Model file for the job. Use its own axes, mm. Round coordinates to 2 decimals unless told otherwise and drop trailing zeros. Order: outer loops, then holes, each group sorted by start corner. A loop starts at its lowest first (then second) coordinate and runs counter-clockwise, first axis right, second up. Notation, with made-up numbers: (4, -17.75) - (23, -17.75) arc R21 cw to (23, -4.75) - close; hole circle Ø10 at (-2.5, 31). An arc over 180 degrees is marked (long way). Put each result on its own line as item: value. Start each with the question number.
Item 1: Saw through at B-B on x = -4.5. List the corners of the cut face in (y, z), plus the area to 3 significant figures.
Item 2: Saw through at A-A on y = 0. List the corners of the cut face in (x, z).
Item 3: Probe probe 1 along Y at (x, z) = (0, 1.05); probe 2 along X at (y, z) = (11, 2.2); probe 3 along X at (y, z) = (-3, 0.7). List the from-to ranges inside material, lowest first.
Item 4: Mould opens along Y. For faces 1 (the face through (63.5, 0, 1)), 2 (the face through (31, 19.939, 1)), 3 (the face through (-3.909, -17.605, 1.288)) say: pulls with the +Y half, pulls with the -Y half, needs draft (parallel to the pull), parting line crosses it, or undercut.
Item 5: Saw through at C-C on z = 1.8. List the corners of the cut face in (x, y).
```python
from build123d import *

# Parameters (mm, degrees)
SKETCH1_R           = 19.939
BOSS_EXTRUDE1_DEPTH = 2.54
SKETCH3_W           = 2.54
SKETCH3_H           = 39.878
BOSS_EXTRUDE2_DEPTH = 63.5
SKETCH2_R           = 18.034
CUT_EXTRUDE1_DEPTH  = 2.54


with BuildPart() as part:
    # Sketch1 → Boss-Extrude1 (new body)
    with BuildSketch(Plane.XY):
        Circle(SKETCH1_R)
    extrude(amount=BOSS_EXTRUDE1_DEPTH)

    # Sketch3 → Boss-Extrude2 (add)
    with BuildSketch(Plane(origin=(0, 0, 0), x_dir=(0, 0, -1), z_dir=(1, 0, 0))):
        with Locations((-1.27, 0)):
            Rectangle(SKETCH3_W, SKETCH3_H)
    extrude(amount=BOSS_EXTRUDE2_DEPTH)

    # Sketch2 → Cut-Extrude1 (cut)
    with BuildSketch(Plane.XY.offset(2.54)):
        Circle(SKETCH2_R)
    extrude(amount=-CUT_EXTRUDE1_DEPTH, mode=Mode.SUBTRACT)


solid = part.part
```
Results found:
1. outline: (-19.42, 0) - (-17.46, 0) - (-17.46, 2.54) - (-19.42, 2.54) - close; (17.46, 0) - (19.42, 0) - (19.42, 2.54) - (17.46, 2.54) - close
1. area: 9.96 mm²
2. outline: (-19.94, 0) - (-18.03, 0) - (-18.03, 2.54) - (-19.94, 2.54) - close; (18.03, 0) - (63.5, 0) - (63.5, 2.54) - (18.03, 2.54) - close
3. probe 1: y = -19.94 to -18.03, 18.03 to 19.94
3. probe 2: x = -16.63 to -14.29, 14.29 to 63.5
3. probe 3: x = -19.71 to -17.78, 17.78 to 63.5
4. face 1: needs draft
4. face 2: pulls with the +Y half
4. face 3: undercut
5. outline: (0, -19.94) - (63.5, -19.94) - (63.5, 19.94) - (0, 19.94) arc R19.94 ccw to start; hole circle Ø36.07 at (0, 0)
